Job drawing, mm, ordinate dimensions from the low corner. One solid piece. A direction names the side the tool comes from. Give positions to 0.01 mm unless a question says otherwise; leave off trailing zeros. Loops run counter-clockwise (first coordinate to the right, second up) from the corner with the lowest first, then second, coordinate; pieces in that order, holes last. Notation, with made-up numbers: M 27,18.25 L 46,18.25 A21 ccw 46,48.25 Z; hole C 11.5,13.5 d2. An arc over 180 degrees is marked long. Put each result on its own line as item: value.
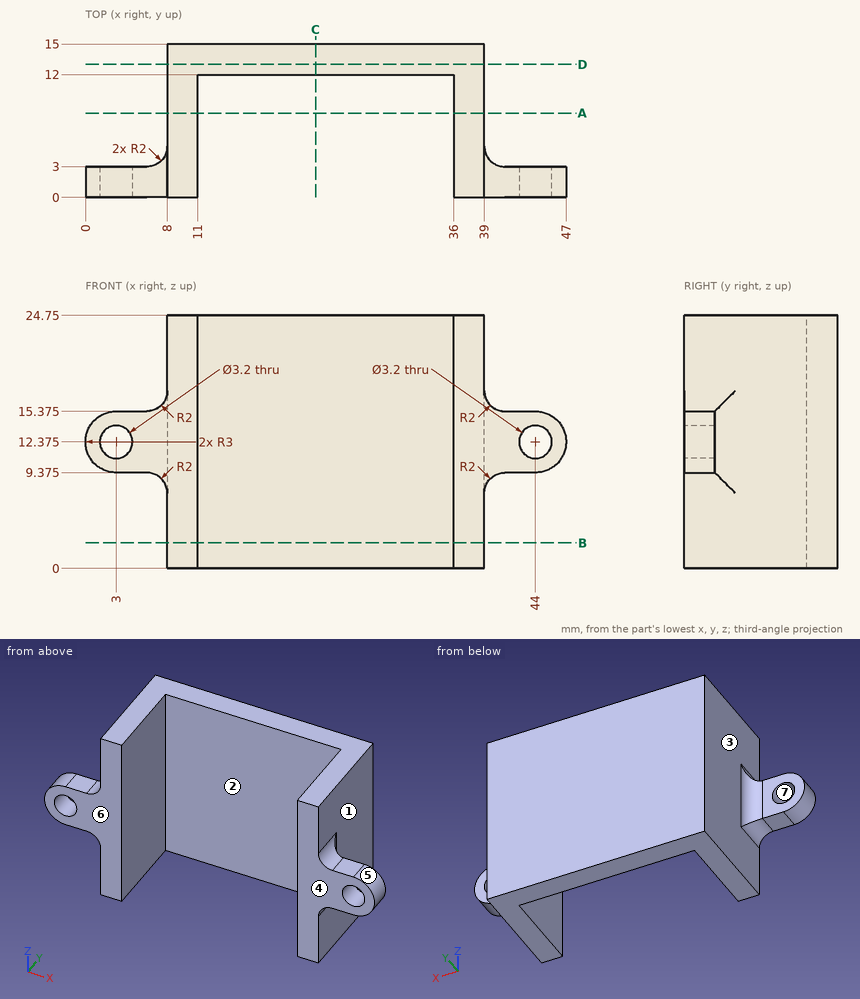
Q1. Slice it at B-B (z = 2.5). List the corners of the cut face in (x, y).
Here are the results:
outline: M 8,0 L 11,0 L 11,12 L 36,12 L 36,0 L 39,0 L 39,15 L 8,15 Z
Q2. Slice it at A-A (y = 8.25). List the corners of the cut face in (x, z).
Here are the results:
outline: M 8,0 L 11,0 L 11,24.75 L 8,24.75 Z; M 36,0 L 39,0 L 39,24.75 L 36,24.75 Z
Q3. Probe line 1 (X direction, y = 2.25, z = 7); line 2 (Z direction, x = 3, y = 0.7) (3 decimals); line 3 (Y direction, x = 19, z = 4). List the from-to ranges inside material, lowest first. Write a range as from..to.
Here are the results:
line 1: 8..11, 36..39
line 2: 9.375..10.775, 13.975..15.375
line 3: 12..15
Q4. Slice it at D-D (y = 13). List the corners of the cut face in (x, z).
Here are the results:
outline: M 8,0 L 39,0 L 39,24.75 L 8,24.75 Z
Q5. Slice it at C-C (x = 22.5). List the corners of the cut face in (y, z), and give its area (4 significant figures).
Here are the results:
outline: M 12,0 L 15,0 L 15,24.75 L 12,24.75 Z
area: 74.25 mm²
Q6. Tool access for the marked faces 1, 2, 3 and 4: list every direction of +Z, -Z, +X, -X, +Y, -Y with a clear straight run to the whole face (end or side of a thin tool).
Here are the results:
face 1: +X, +Y
face 2: +Z, -Z, -Y
face 3: -X, +Y
face 4: +Z, -Z, +X, -X, -Y
Q7. Mould opens along X. For the marked faces 5, 6 and 7 say: pulls with the +X half, pulls with the -X half, needs draft (parallel to the pull), parting line crosses it, or undercut.
Here are the results:
face 5: pulls with the +X half
face 6: needs draft
face 7: undercut
Q8. Drop flat-ended pins along their axis: pin 1 Ø1.5 at (y, z) = (2.5, 5.5) entering from +X; pin 2 Ø1.8 at (x, z) = (42.5, 14) entering from +Y; pin 3 Ø4.5 at (y, z) = (5, 9.5) entering from +X. Give the stop position or say it passes through.
Here are the results:
pin 1: x = 39
pin 2: y = 3
pin 3: x = 46.37
